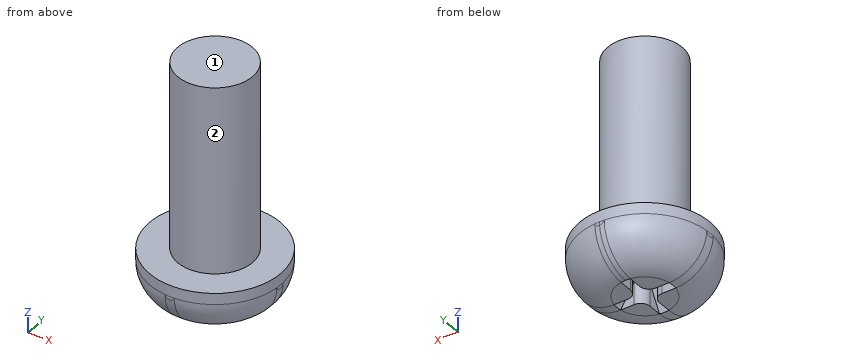
Autodesk Inventor part; units mm, degrees
ref_plane "YZ Plane" through (0, 0, 0) normal (1, 0, 0) x (0, 1, 0)
ref_plane "XZ Plane" through (0, 0, 0) normal (0, 1, 0) x (-1, 0, 0)
ref_plane "XY Plane" through (0, 0, 0) normal (0, 0, 1) x (1, 0, 0)
sketch "スケッチ1" plane through (0, 0, 0) normal (1, 0, 0) x (0, 1, 0)
  line L0 (0, 6.3) -> (0, 0)
  line L1 (0, 0) -> (0.75, 0)
  line L2 (1.75, 1) -> (1.75, 1.3)
  line L3 (1.75, 1.3) -> (1, 1.3)
  line L4 (1, 1.3) -> (1, 6.3)
  line L5 (1, 6.3) -> (0, 6.3)
  line L6 (0.75, 0) -> (0, 1.3)
  arc A0 (0.75, 0) -> (1.75, 1) centre (0.75, 1) ccw
  line L7 (0.75, 0) -> (1.75, 0)
  line L8 (1.75, 0) -> (1.75, 1)
  dimension "d2" = 1.3
  dimension "d10" = 5
  dimension "d11" = 2
  dimension "d12" = 3.5
  dimension "d14" = 1
revolve "回転1" add sketch "スケッチ1" angle 360 about axis through (0, 0, 6.3) along (0, 0, -1) contours L5 L4 L3 L2 A0 L6 L0
thread "ねじ1"
sketch "スケッチ2" plane through (0, 0, 1.3) normal (0, 0, 1) x (1, 0, 0)
  line L0 (0.125, -1.7455) -> (-0.125, -1.7455)
  line L1 (-0.125, -1.7455) -> (-0.125, -0.375)
  line L2 (-0.125, 1.7455) -> (0.125, 1.7455)
  line L3 (0.125, 1.7455) -> (0.125, 0.375)
  line L4 (0.125, -1.7455) -> (-0.125, 1.7455) construction
  line L5 (-0.125, -1.7455) -> (0.125, 1.7455) construction
  line L6 (-1.7455, 0.125) -> (-0.375, 0.125)
  line L7 (1.7455, 0.125) -> (1.7455, -0.125)
  line L8 (1.7455, -0.125) -> (0.375, -0.125)
  line L9 (-1.7455, -0.125) -> (-1.7455, 0.125)
  line L10 (-1.7455, 0.125) -> (1.7455, -0.125) construction
  line L11 (1.7455, 0.125) -> (-1.7455, -0.125) construction
  line L12 (0.125, -0.375) -> (0.125, -1.7455)
  line L13 (0.375, 0.125) -> (1.7455, 0.125)
  line L14 (-0.375, -0.125) -> (-1.7455, -0.125)
  line L15 (-0.125, 0.375) -> (-0.125, 1.7455)
  arc A0 (0.375, -0.125) -> (0.125, -0.375) centre (0.375, -0.375) ccw
  arc A1 (0.125, 0.375) -> (0.375, 0.125) centre (0.375, 0.375) ccw
  arc A2 (-0.375, 0.125) -> (-0.125, 0.375) centre (-0.375, 0.375) ccw
  arc A3 (-0.125, -0.375) -> (-0.375, -0.125) centre (-0.375, -0.375) ccw
  circle A4 centre (0, 0) radius 1.75
  line L16 (0, 1.75) -> (0, -1.75) construction
  line L17 (1.7455, 0) -> (-1.7455, 0) construction
  point P0 (-0.3339, -0.2226)
  point P1 (-0.3339, 0.2226)
  point P2 (0.3339, 0.2226)
  point P3 (0.3339, -0.2226)
  point P4 (0, 0)
  dimension "d18" = 0.25
  dimension "d19" = 0.25
  dimension "d20" = 0.25
extrude "押し出し2" add sketch "スケッチ2" against normal blind 1.3 contours A4 L0 | L12 A0 L8 A4 | A4 L14 A3 L1 | L7 A4 | A4 L9 | L13 A1 L3 A4 | A4 L15 A2 L6 | L2 A4
revolve "回転2" cut sketch "スケッチ1" angle 360 about axis through (0, 0, 6.3) along (0, 0, -1) contours A0 L8 L7
equation "\"d19\" = d20"
equation "\"d20\" = d18"
properties part number "U-0205" material "Stainless Steel"
The listing builds one solid part. Answer for the finished solid, in the listing's coordinates (mm). Face numbers are marked on the shaded views. A direction names the side the tool comes from. Coordinates: 2 decimals unless noted, no trailing zeros. Loops run counter-clockwise (first coordinate to the right, second up) from the corner with the lowest first, then second, coordinate; pieces in that order, holes last.
1) Find section A-A on z = 3. Write down the section's boundary in (x, y).
2) Flat-ended cylindrical pins translate along their axes: pin 1 Ø1 at (y, z) = (-0.5, 3) entering from +X; pin 2 Ø1.5 at (x, z) = (1, 1.5) entering from +Y. Find the tip coordinate at first contact, or state that the pin passes through.
3) A tool of negligible diameter and unlimited length cuts with its end or side. For the marked faces 1 and 2, from which of +Z, -Z, +X, -X, +Y, -Y can it reach the whole face along a straight path? Write none if from no direction.
4) Find the intervals of material crossed by L1, parallel to Z at x = -0.1, y = -0.3; L2, parallel to Z at x = 0.8, y = 0.05; L3, parallel to X at y = -0.05, z = 3, in increasing order.
Values:
1. outline: circle Ø2 at (0, 0)
2. pin 1: stops at x = 1
2. pin 2: stops at y = 1.73
3. face 1: +Z, +X, -X, +Y, -Y
3. face 2: +Z
4. L1: z = 0.75 to 6.3
4. L2: z = 0 to 6.3
4. L3: x = -1 to 1
